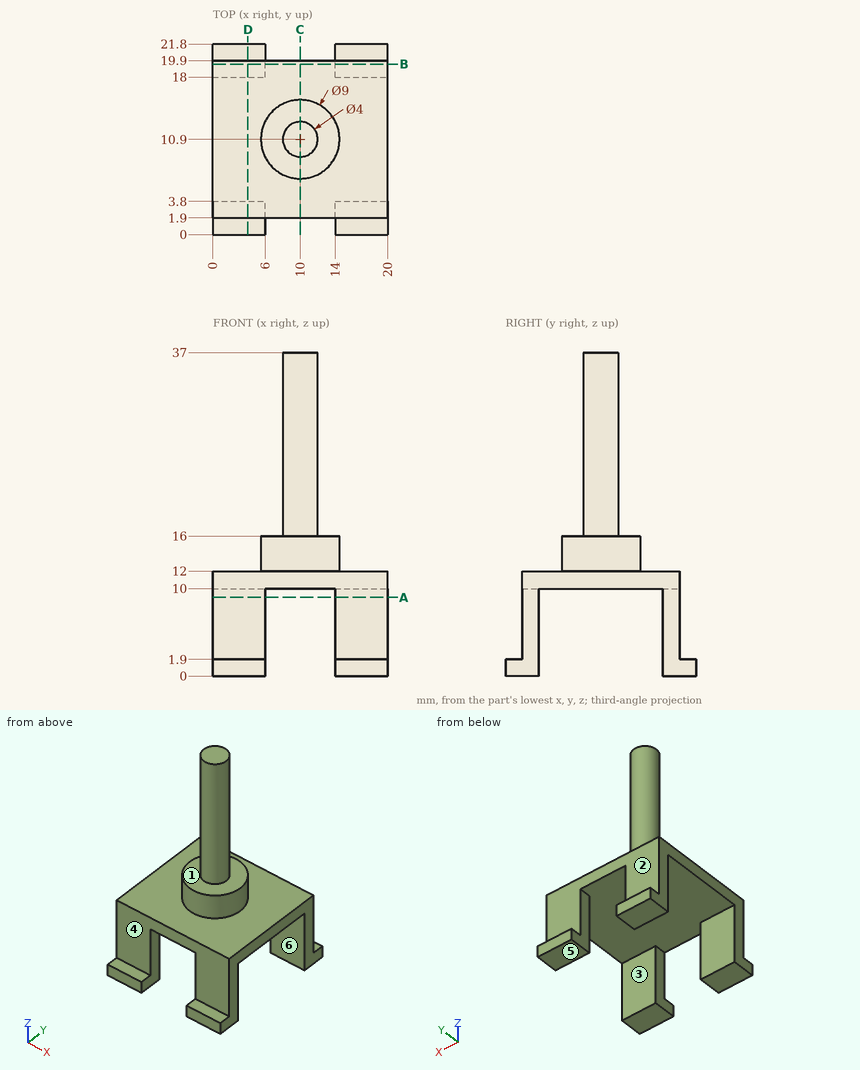
Part print with two shaded views. Sizes in mm from the minimum x, y, z corner. A direction names the side the tool comes from. Give positions to 0.01 mm unless a question says otherwise; leave off trailing zeros. Order: outer loops, then holes, each group sorted by start corner. A loop starts at its lowest first (then second) coordinate and runs counter-clockwise, first axis right, second up.
1) 3-axis set-ups, long thin cutter, end or side, ignore diameter. For the marked faces 1, 2 and 3: which of +Z, -Z, +X, -X, +Y, -Y reach the whole face in a straight line?
2) Pin check, flat tips, straight feed: pin 1 (3 mm diameter, centred on x = 15.5, z = 4, fed in from -Y); pin 2 (1 mm diameter, centred on x = 17, y = 0.5, fed in from +Z); pin 3 (5 mm diameter, centred on x = 12.5, z = 17.5, fed in from -Y); pin 4 (4 mm diameter, centred on x = 2.5, z = 14.5, fed in from -Y). Stop position of each tip, or through.
3) Saw through at A-A, the plane z = 9. Write the cut outline in (x, y), then the cut area to 3 significant figures.
4) Saw through at B-B, the plane y = 19.5. Write the cut outline in (x, z).
5) Mould opens along Y. For the marked faces 4, 5 and 6 say: +Y half, -Y half, draft (parallel to the pull), parting line (faces both ways), or undercut.
6) Saw through at D-D, the plane x = 4. Write the cut outline in (y, z).
7) Wall check: probe 1 along Y at (x, z) = (16.5, 5); probe 2 along Z at (x, y) = (17.5, 16.25); probe 3 along Y at (x, z) = (10, 11.5). Give the ranges that are in metal, low to high.
8) Saw through at C-C, the plane x = 10. Write the cut outline in (y, z).
Computed:
1. face 1: +Z
1. face 2: +Z, +X, -X, +Y
1. face 3: -Z, +X, -X
2. pin 1: stops at y = 1.9
2. pin 2: stops at z = 1.9
2. pin 3: stops at y = 6.43
2. pin 4: passes through
3. outline: (0, 1.9) - (6, 1.9) - (6, 3.8) - (0, 3.8) - close; (0, 18) - (6, 18) - (6, 19.9) - (0, 19.9) - close; (14, 1.9) - (20, 1.9) - (20, 3.8) - (14, 3.8) - close; (14, 18) - (20, 18) - (20, 19.9) - (14, 19.9) - close
3. area: 45.6 mm2
4. outline: (0, 0) - (6, 0) - (6, 10) - (14, 10) - (14, 0) - (20, 0) - (20, 12) - (0, 12) - close
5. face 4: -Y half
5. face 5: draft
5. face 6: undercut
6. outline: (0, 0) - (3.8, 0) - (3.8, 10) - (18, 10) - (18, 0) - (21.8, 0) - (21.8, 1.9) - (19.9, 1.9) - (19.9, 12) - (1.9, 12) - (1.9, 1.9) - (0, 1.9) - close
7. probe 1: y = 1.9 to 3.8, 18 to 19.9
7. probe 2: z = 10 to 12
7. probe 3: y = 1.9 to 19.9
8. outline: (1.9, 10) - (19.9, 10) - (19.9, 12) - (15.4, 12) - (15.4, 16) - (12.9, 16) - (12.9, 37) - (8.9, 37) - (8.9, 16) - (6.4, 16) - (6.4, 12) - (1.9, 12) - close
